```python
from build123d import *

# Parameters (mm, degrees)
CHAMFER1_SIZE      = 0.25
FILLET1_R          = 0.2
CUT_EXTRUDE1_DEPTH = 2
FILLET2_R          = 0.1


with BuildPart() as part:
    # Sketch1 → Revolve1 (revolve)
    with BuildSketch(Plane.XY):
        Polygon((0, -7), (-1.5, -7), (-1.5, -3), (-2.75, -3), (-2.75, 0), (0, 0), align=None)
    revolve(axis=Axis((0, 0, 0), (0, -1, 0)))

    # Chamfer1
    chamfer1_edges = [part.edges().sort_by_distance(p)[0] for p in [
        (1.5, -3, 0),
        (1.5, -7, 0),
    ]]
    chamfer(chamfer1_edges, length=CHAMFER1_SIZE)

    # Fillet1
    fillet1_edges = [part.edges().sort_by_distance(p)[0] for p in [
        (2.75, 0, 0),
    ]]
    fillet(fillet1_edges, radius=FILLET1_R)

    # Sketch2 → Cut-Extrude1 (cut)
    with BuildSketch(Plane(origin=(0, 0, 0), x_dir=(1, 0, 0), z_dir=(0, 1, 0))):
        Polygon((0, 1.443375673), (-1.25, 0.721687836), (-1.25, -0.721687836), (0, -1.443375673), (1.25, -0.721687836), (1.25, 0.721687836), align=None)
    extrude(amount=-CUT_EXTRUDE1_DEPTH, mode=Mode.SUBTRACT)

    # Fillet2
    fillet2_edges = [part.edges().sort_by_distance(p)[0] for p in [
        (0.625, -2, -1.082531755),
        (1.25, -2, 0),
        (0.625, -2, 1.082531755),
        (-0.625, -2, 1.082531755),
        (-1.25, -2, 0),
        (-0.625, -2, -1.082531755),
        (0.625, 0, -1.082531755),
        (-0.625, 0, -1.082531755),
        (-1.25, 0, 0),
        (-0.625, 0, 1.082531755),
        (0.625, 0, 1.082531755),
        (1.25, 0, 0),
    ]]
    fillet(fillet2_edges, radius=FILLET2_R)


solid = part.part
```
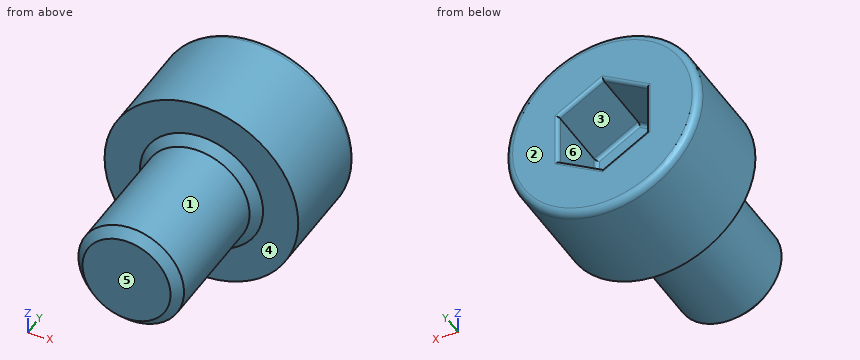
The model under review builds one solid part; all positions refer to its coordinate system, in mm. Face numbers are marked on the shaded views. A direction names the side the tool comes from. Round coordinates to 2 decimals unless told otherwise and drop trailing zeros. Order: outer loops, then holes, each group sorted by start corner. A loop starts at its lowest first (then second) coordinate and runs counter-clockwise, first axis right, second up. Notation, with made-up numbers: (6, 72) -> (22, 72) arc R21 cw to (22, 97) -> close; hole circle Ø1 at (43, -13.75). An arc over 180 degrees is marked (long way). One line per item, written item: value. Start each with the question number.
Q1. Wall thickness on line 1 (Y direction, x = 1.4, z = -1.9); line 2 (Z direction, x = -1, y = -0.5); line 3 (X direction, y = -0.25, z = -1.2): over which ranges is each line inside the solid? List them lowest first.
Q2. Take a section at B-B (z = 0). Write out the cut boundary in (x, y), and give its area (3 significant figures).
Q3. Take a section at C-C (y = -6). Write out the cut boundary in (x, z).
Q4. Take a section at A-A (y = -1). Write out the cut boundary in (x, z).
Q5. Machinability: for the marked faces 4, 5 and 6, which of the approach directions +Z, -Z, +X, -X, +Y, -Y give a long, thin tool a straight path to every point of the face, cutting with its end or side? Answer none if there is none.
Q6. Mouldability with a two-part tool opening along X and no side actions: class the marked faces 1, 2 and 3 as released by +X, released by -X, zero draft, split by the parting line, or undercut.
Reported:
1. line 1: y = -3 to 0
1. line 2: z = -2.56 to -0.87, 0.87 to 2.56
1. line 3: x = -2.47 to -0.42, 0.42 to 2.47
2. outline: (-2.75, -3) -> (-1.75, -3) -> (-1.5, -3.25) -> (-1.5, -6.75) -> (-1.25, -7) -> (1.25, -7) -> (1.5, -6.75) -> (1.5, -3.25) -> (1.75, -3) -> (2.75, -3) -> (2.75, -0.2) arc R0.2 ccw to (2.55, 0) -> (1.35, 0) arc R0.1 ccw to (1.25, -0.1) -> (1.25, -1.9) arc R0.1 cw to (1.15, -2) -> (-1.15, -2) arc R0.1 cw to (-1.25, -1.9) -> (-1.25, -0.1) arc R0.1 ccw to (-1.35, 0) -> (-2.55, 0) arc R0.2 ccw to (-2.75, -0.2) -> close
2. area: 23.5 mm2
3. outline: circle Ø3 at (0, 0)
4. outline: circle Ø5.5 at (0, 0); hole (-1.25, -0.72) -> (0, -1.44) -> (1.25, -0.72) -> (1.25, 0.72) -> (0, 1.44) -> (-1.25, 0.72) -> close
5. face 4: -Y
5. face 5: +Z, -Z, +X, -X, -Y
5. face 6: +Y
6. face 1: split by the parting line
6. face 2: zero draft
6. face 3: undercut
